Could you check a few things on this drawing? It's one solid part, dimensions in mm from its lowest x, y, z. Give positions to 0.01 mm unless a question says otherwise; leave off trailing zeros. Order: outer loops, then holes, each group sorted by start corner. A loop starts at its lowest first (then second) coordinate and runs counter-clockwise, first axis right, second up. Notation, with made-up numbers: (80, 72.25) - (130, 72.25) arc R30 ccw to (130, 106.25) - close; hole circle Ø11 at (4.25, 16.25). An arc over 180 degrees is marked (long way). Answer as CSV lines item,"result".
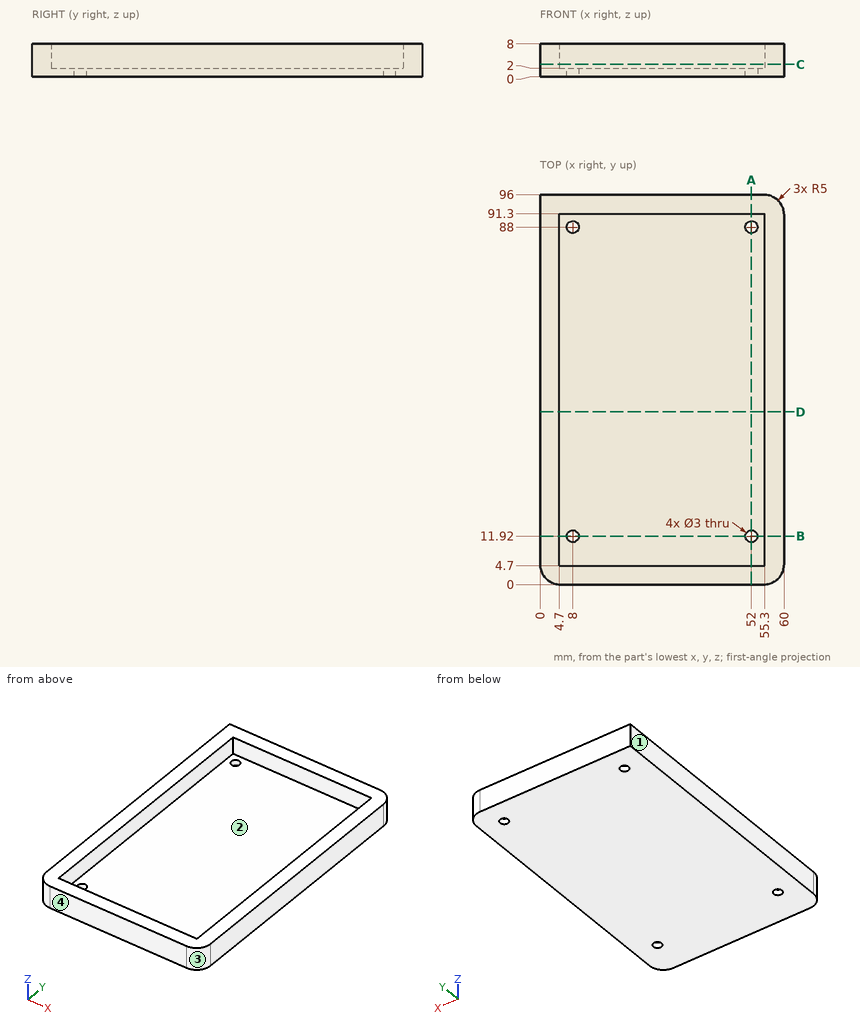
1) I want a section at C-C on z = 3. Write out the boundary of the cut face in (x, y).
Answer block:
outline,"(0, 5) arc R5 ccw to (5, 0) - (55, 0) arc R5 ccw to (60, 5) - (60, 91) arc R5 ccw to (55, 96) - (0, 96) - close; hole (4.7, 4.7) - (55.3, 4.7) - (55.3, 91.3) - (4.7, 91.3) - close"
2) I want a section at D-D on y = 42.5. Write out the boundary of the cut face in (x, z), plus the area to 3 significant figures.
Answer block:
outline,"(0, 0) - (60, 0) - (60, 8) - (55.3, 8) - (55.3, 2) - (4.7, 2) - (4.7, 8) - (0, 8) - close"
area,"176 mm2"
3) I'm going to push a flat-ended pin straight in: P1, Ø5, axis at x = 52, y = 88, coming from the +Z side. Where does the tip first touch, or does it pass through?
Answer block:
P1,"z = 2"
4) I want a section at B-B on y = 11.92. Write out the boundary of the cut face in (x, z).
Answer block:
outline,"(0, 0) - (6.5, 0) - (6.5, 2) - (4.7, 2) - (4.7, 8) - (0, 8) - close; (9.5, 0) - (50.5, 0) - (50.5, 2) - (9.5, 2) - close; (53.5, 0) - (60, 0) - (60, 8) - (55.3, 8) - (55.3, 2) - (53.5, 2) - close"
5) If we mould it in two halves opening along X, with no side actions, what happens to the marked faces 1, 2, 3 and 4? For each: +X half, -X half, draft (parallel to the pull), parting line (faces both ways), or undercut.
Answer block:
face 1,"-X half"
face 2,"undercut"
face 3,"+X half"
face 4,"draft"
6) I need wall thicknesses on line 1 along Y through (x, z) = (52, 1.05); line 2 along Y through (x, z) = (26.5, 4); line 3 along X through (y, z) = (66, 7.25). Which ranges of each line are inside material? Lowest first, please. Write a range as [from, to].
Answer block:
line 1,"[0, 10.42], [13.42, 86.5], [89.5, 96]"
line 2,"[0, 4.7], [91.3, 96]"
line 3,"[0, 4.7], [55.3, 60]"
7) I want a section at A-A on x = 52. Write out the boundary of the cut face in (y, z), plus the area to 3 significant figures.
Answer block:
outline,"(0, 0) - (10.42, 0) - (10.42, 2) - (4.7, 2) - (4.7, 8) - (0, 8) - close; (13.42, 0) - (86.5, 0) - (86.5, 2) - (13.42, 2) - close; (89.5, 0) - (96, 0) - (96, 8) - (91.3, 8) - (91.3, 2) - (89.5, 2) - close"
area,"236 mm2"
